```python
from build123d import *

# Parameters (mm, degrees)
SKETCH_1_R      = 1.5
SKETCH_1_R_2    = 1.55
SKETCH_1_R_3    = 10
SKETCH_1_W      = 30
SKETCH_1_H      = 10
EXTRUDE_1_DEPTH = 3.5
FILLET_1_R      = 5
SKETCH_2_W      = 20
SKETCH_2_H      = 20
SKETCH_2_R      = 1.5
EXTRUDE_2_DEPTH = 48
FILLET_2_R      = 5


with BuildPart() as part:
    # 草图1 → 凸台-拉伸1 (new body)
    with BuildSketch(Plane(origin=(0, 0, 0), x_dir=(1, 0, 0), z_dir=(0, 1, 0))):
        Polygon((-100, 100), (100, 100), (100, -32.687538375), (100, -80.687538375), (100, -100), (-100, -100), (-100, -80.687538375), (-100, -32.687538375), align=None)
        with Locations(Location((-55, 10, 0), (0, 0, 270))):
            Circle(SKETCH_1_R, mode=Mode.SUBTRACT)
        with Locations(Location((-55, -71, 0), (0, 0, 270))):
            Circle(SKETCH_1_R, mode=Mode.SUBTRACT)
        with Locations(Location((55, -71, 0), (0, 0, 90))):
            Circle(SKETCH_1_R, mode=Mode.SUBTRACT)
        with Locations(Location((55, 10, 0), (0, 0, 90))):
            Circle(SKETCH_1_R, mode=Mode.SUBTRACT)
        with Locations(Location((60, 94, 0), (0, 0, 270))):
            Circle(SKETCH_1_R_2, mode=Mode.SUBTRACT)
        with Locations(Location((60, -94, 0), (0, 0, 270))):
            Circle(SKETCH_1_R_2, mode=Mode.SUBTRACT)
        with Locations(Location((94, 20, 0), (0, 0, 270))):
            Circle(SKETCH_1_R_2, mode=Mode.SUBTRACT)
        with Locations(Location((94, -20, 0), (0, 0, 90))):
            Circle(SKETCH_1_R_2, mode=Mode.SUBTRACT)
        with Locations(Location((-60, -94, 0), (0, 0, 90))):
            Circle(SKETCH_1_R_2, mode=Mode.SUBTRACT)
        with Locations(Location((-94, -20, 0), (0, 0, 270))):
            Circle(SKETCH_1_R_2, mode=Mode.SUBTRACT)
        with Locations(Location((-94, 20, 0), (0, 0, 90))):
            Circle(SKETCH_1_R_2, mode=Mode.SUBTRACT)
        with Locations(Location((-60, 94, 0), (0, 0, 90))):
            Circle(SKETCH_1_R_2, mode=Mode.SUBTRACT)
        with Locations(Location((0, 29.5, 0), (0, 0, 270))):
            Circle(SKETCH_1_R, mode=Mode.SUBTRACT)
        with Locations(Location((20.859650045, 20.859650045, 0), (0, 0, 270))):
            Circle(SKETCH_1_R, mode=Mode.SUBTRACT)
        with Locations(Location((29.5, 0, 0), (0, 0, 270))):
            Circle(SKETCH_1_R, mode=Mode.SUBTRACT)
        with Locations(Location((20.859650045, -20.859650045, 0), (0, 0, 270))):
            Circle(SKETCH_1_R, mode=Mode.SUBTRACT)
        with Locations(Location((0, -29.5, 0), (0, 0, 270))):
            Circle(SKETCH_1_R, mode=Mode.SUBTRACT)
        with Locations(Location((-20.859650045, -20.859650045, 0), (0, 0, 270))):
            Circle(SKETCH_1_R, mode=Mode.SUBTRACT)
        with Locations(Location((-29.5, 0, 0), (0, 0, 270))):
            Circle(SKETCH_1_R, mode=Mode.SUBTRACT)
        with Locations(Location((-20.859650045, 20.859650045, 0), (0, 0, 270))):
            Circle(SKETCH_1_R, mode=Mode.SUBTRACT)
        with Locations(Location((70, 50, 0), (0, 0, 270))):
            Circle(SKETCH_1_R_3, mode=Mode.SUBTRACT)
        with Locations((15, -45)):
            Rectangle(SKETCH_1_W, SKETCH_1_H, mode=Mode.SUBTRACT)
    extrude(amount=EXTRUDE_1_DEPTH)

    # 圆角1
    fillet_1_edges = [part.edges().sort_by_distance(p)[0] for p in [
        (-100, 1.75, -100),
        (100, 1.75, -100),
        (100, 1.75, 100),
        (-100, 1.75, 100),
    ]]
    fillet(fillet_1_edges, radius=FILLET_1_R)

    # 草图2 → 凸台-拉伸2 (add)
    # profile 1 of 4: a face of its own
    with BuildSketch(Plane(origin=(0, 3.5, 0), x_dir=(1, 0, 0), z_dir=(0, 1, 0))):
        with Locations((-90, 90)):
            Rectangle(SKETCH_2_W, SKETCH_2_H)
        with Locations(Location((-90, 90, 0), (0, 0, 270))):
            Circle(SKETCH_2_R, mode=Mode.SUBTRACT)
    # profile 2 of 4: a face of its own
    with BuildSketch(Plane(origin=(0, 3.5, 0), x_dir=(1, 0, 0), z_dir=(0, 1, 0))):
        with Locations((90, 90)):
            Rectangle(SKETCH_2_W, SKETCH_2_H)
        with Locations(Location((90, 90, 0), (0, 0, 90))):
            Circle(SKETCH_2_R, mode=Mode.SUBTRACT)
    # profile 3 of 4: a face of its own
    with BuildSketch(Plane(origin=(0, 3.5, 0), x_dir=(1, 0, 0), z_dir=(0, 1, 0))):
        with Locations((90, -90)):
            Rectangle(SKETCH_2_W, SKETCH_2_H)
        with Locations(Location((90, -90, 0), (0, 0, 270))):
            Circle(SKETCH_2_R, mode=Mode.SUBTRACT)
    # profile 4 of 4: a face of its own
    with BuildSketch(Plane(origin=(0, 3.5, 0), x_dir=(1, 0, 0), z_dir=(0, 1, 0))):
        with Locations((-90, -90)):
            Rectangle(SKETCH_2_W, SKETCH_2_H)
        with Locations(Location((-90, -90, 0), (0, 0, 90))):
            Circle(SKETCH_2_R, mode=Mode.SUBTRACT)
    extrude(amount=EXTRUDE_2_DEPTH)

    # 圆角2
    fillet_2_edges = [part.edges().sort_by_distance(p)[0] for p in [
        (100, 27.5, 100),
        (100, 27.5, -100),
        (-100, 27.5, -100),
        (-100, 27.5, 100),
    ]]
    fillet(fillet_2_edges, radius=FILLET_2_R)


solid = part.part
```
Here's how the part is built. I have some questions about the finished solid (model axes, mm). A direction names the side the tool comes from. Coordinates: 2 decimals unless noted, no trailing zeros. Order: outer loops, then holes, each group sorted by start corner. A loop starts at its lowest first (then second) coordinate and runs counter-clockwise, first axis right, second up. Notation, with made-up numbers: (38.25, 28) - (48.25, 28) arc R16 cw to (48.25, 59) - close; hole circle Ø4 at (-36.5, 43). An arc over 180 degrees is marked (long way). One line per question, with ' | ' between items.
(1) If I drill on L1, parallel to X at y = 2, z = 94; L2, parallel to X at y = 28.5, z = -90; L3, parallel to X at y = 1.55, z = 20, over which ranges is the centre line in solid material (lowest first)?
Report:
L1: x = -100 to -61.55, -58.45 to 58.45, 61.55 to 100 | L2: x = -100 to -91.5, -88.5 to -80, 80 to 88.5, 91.5 to 100 | L3: x = -100 to -95.55, -92.45 to -22.09, -19.63 to 19.63, 22.09 to 92.45, 95.55 to 100
(2) If we mould it in two halves opening along X, with no side actions, what happens to faces 1 (the cylindrical face through (98, 2, -99)), 2 (the flat face through (-90, 51.5, 88)), 3 (the flat face through (-100, 1, 0)), 4 (the cylindrical face through (76.76, 1.73, -57.37))? For each: pulls with the +X half, pulls with the -X half, needs draft (parallel to the pull), parting line crosses it, or undercut.
Report:
face 1: pulls with the +X half | face 2: needs draft | face 3: pulls with the -X half | face 4: undercut
(3) Suppose I cut it at C-C on z = -50. List the corners of the cut face in (x, y) for me, and give its area (3 significant figures).
Report:
outline: (-100, 0) - (60, 0) - (60, 3.5) - (-100, 3.5) - close; (80, 0) - (100, 0) - (100, 3.5) - (80, 3.5) - close | area: 630 mm2
(4) Suppose I cut it at A-A on z = 44. List the corners of the cut face in (x, y) for me, and give its area (3 significant figures).
Report:
outline: (-100, 0) - (0, 0) - (0, 3.5) - (-100, 3.5) - close; (30, 0) - (100, 0) - (100, 3.5) - (30, 3.5) - close | area: 595 mm2
(5) Suppose I cut it at D-D on z = -4.5. List the corners of the cut face in (x, y) for me.
Report:
outline: (-100, 0) - (100, 0) - (100, 3.5) - (-100, 3.5) - close
(6) Suppose I cut it at B-B on y = 28. List the corners of the cut face in (x, z) for me, and give its area (3 significant figures).
Report:
outline: (-100, -95) arc R5 ccw to (-95, -100) - (-80, -100) - (-80, -80) - (-100, -80) - close; (-100, 80) - (-80, 80) - (-80, 100) - (-95, 100) arc R5 ccw to (-100, 95) - close; (80, -100) - (95, -100) arc R5 ccw to (100, -95) - (100, -80) - (80, -80) - close; (80, 80) - (100, 80) - (100, 95) arc R5 ccw to (95, 100) - (80, 100) - close; hole circle Ø3 at (-90, -90); hole circle Ø3 at (-90, 90); hole circle Ø3 at (90, -90); hole circle Ø3 at (90, 90) | area: 1,550 mm2
(7) For faces 5 (the flat face through (-80, 27, -90)), 6 (the flat face through (0, 1, -100)), 7 (the flat face through (90, 27, 80)), which set-ups out of +Z, -Z, +X, -X, +Y, -Y let a thin tool reach every point of the face, with its end or its side?
Report:
face 5: +Z, -Z, +Y | face 6: -Z, +X, -X, +Y, -Y | face 7: +X, -X, +Y
(8) Will this pin go through, and if not, where does the flat tip stop? pin 1 (6 mm diameter, centred on x = 52, z = -26, fed in from +Y).
Report:
pin 1: stops at y = 3.5
